Input: part model. Units: mm. Frame: model coordinates. Round coordinates to 2 decimals unless told otherwise and drop trailing zeros. Write each loop counter-clockwise with the first axis right and the second up, starting at its lowest first coordinate (ties: lowest second). Pieces come first, ordered by that corner, then holes. Notation, with made-up numbers: (-31.75, 60) - (21.25, 60) arc R24 ccw to (21.25, 97) - close; hole circle Ø9 at (38, 87). An arc over 180 degrees is marked (long way). Use one line per item in the form item = value.
```python
from build123d import *

# Parameters (mm, degrees)
SKIZZE1_R                       = 2.5
AUFSATZ_LINEAR_AUSTRAGEN1_DEPTH = 2
SKIZZE2_W                       = 78
SKIZZE2_H                       = 1
SCHNITT_LINEAR_AUSTRAGEN1_DEPTH = 1


with BuildPart() as part:
    # Skizze1 → Aufsatz-Linear austragen1 (new body)
    with BuildSketch(Plane(origin=(0, 0, 0), x_dir=(1, 0, 0), z_dir=(0, 1, 0))):
        with BuildLine():
            Line((0, 0), (78, 0))
            ThreePointArc((78, 0), (95.649655435, 29), (78, 58))
            Line((78, 58), (0, 58))
            Line((0, 58), (0, 0))
        make_face()
        with Locations((88, 29)):
            Circle(SKIZZE1_R, mode=Mode.SUBTRACT)
    extrude(amount=AUFSATZ_LINEAR_AUSTRAGEN1_DEPTH)

    # Skizze2 → Schnitt-Linear austragen1 (cut)
    with BuildSketch(Plane(origin=(0, 2, 0), x_dir=(1, 0, 0), z_dir=(0, 1, 0))):
        with Locations((39, 57.5)):
            Rectangle(SKIZZE2_W, SKIZZE2_H)
        with Locations((39, 0.5)):
            Rectangle(SKIZZE2_W, SKIZZE2_H)
    extrude(amount=-SCHNITT_LINEAR_AUSTRAGEN1_DEPTH, mode=Mode.SUBTRACT)


solid = part.part
```
(1) Draft query along X for faces 1 (the face through (95.646, 0.986, -28.5)), 2 (the face through (86.16, 0.99, -30.69)), 3 (the face through (47, 0, -29)). Return one class per face: released by +X, released by -X, zero draft, split by the parting line, or undercut.
Derived:
face_1 = released by +X
face_2 = undercut
face_3 = zero draft
(2) Material intervals for L1, parallel to X at y = 1, z = -29; L2, parallel to Z at x = 54.5, y = 1.5; L3, parallel to Z at x = 88, y = 1.6, sorted ascending.
Derived:
L1 = 0 to 85.5, 90.5 to 95.65
L2 = -57 to -1
L3 = -50 to -31.5, -26.5 to -8
(3) Cut plane B-B on z = -29. Output: boundary loops of the cut face in (x, y), then the cut area to 3 significant figures.
Derived:
outline = (0, 0) - (85.5, 0) - (85.5, 2) - (0, 2) - close; (90.5, 0) - (95.65, 0) - (95.65, 2) - (90.5, 2) - close
area = 181 mm^2
(4) Cut plane D-D on x = 40. Output: boundary loops of the cut face in (y, z).
Derived:
outline = (0, -58) - (1, -58) - (1, -57) - (2, -57) - (2, -1) - (1, -1) - (1, 0) - (0, 0) - close
(5) Cut plane A-A on x = 88. Output: boundary loops of the cut face in (y, z).
Derived:
outline = (0, -50) - (2, -50) - (2, -31.5) - (0, -31.5) - close; (0, -26.5) - (2, -26.5) - (2, -8) - (0, -8) - close
(6) Cut plane C-C on y = 1.4. Output: boundary loops of the cut face in (x, z), then the cut area to 3 significant figures.
Derived:
outline = (0, -57) - (78, -57) - (78, -58) arc R32.65 ccw to (78, 0) - (78, -1) - (0, -1) - close; hole circle Ø5 at (88, -29)
area = 5,080 mm^2
(7) First-contact query: pin 1 Ø1 at (y, z) = (1.5, -9) entering from +X; pin 2 Ø0.5 at (x, y) = (35, 1.5) entering from -Z. Flat tips, straight axial feed; report the tip coordinate or a pass-through.
Derived:
pin_1 = 89.19
pin_2 = -57
